```python
from build123d import *

# Parameters (mm, degrees)
EXTRUDE_1_DEPTH = 3
FILLET_1_R      = 2.032


with BuildPart() as part:
    # 스케치1 → 보스-돌출1 (new body)
    with BuildSketch(Plane.XY):
        with BuildLine():
            Line((-22.703212056, -30.53470544), (-22.703212056, -27.53470544))
            Line((-22.703212056, -27.53470544), (-19.808212056, -27.53470544))
            Line((-19.808212056, -27.53470544), (-19.808212056, -30.53470544))
            ThreePointArc((-19.808212056, -30.53470544), (-17.458089238, -27.052134486), (-19.755712056, -23.53470544))
            ThreePointArc((-19.755712056, -23.53470544), (-16.806747664, -15.831278272), (-10.426669431, -10.603106234))
            ThreePointArc((-10.426669431, -10.603106234), (-4.615473218, -6.174719455), (-1.296316018, 0.334028993))
            ThreePointArc((-1.296316018, 0.334028993), (-1.766656874, 1.136185733), (-2.575803416, 0.677974178))
            ThreePointArc((-2.575803416, 0.677974178), (-5.721510813, -5.168139004), (-11.025821999, -9.160230838))
            ThreePointArc((-11.025821999, -9.160230838), (-18.562919164, -14.982954912), (-22.755712056, -23.53470544))
            ThreePointArc((-22.755712056, -23.53470544), (-25.053334873, -27.052134486), (-22.703212056, -30.53470544))
        make_face()
    extrude(amount=EXTRUDE_1_DEPTH)

    # 필렛1
    fillet_1_edges = [part.edges().sort_by_distance(p)[0] for p in [
        (-22.755712056, -23.53470544, 1.5),
        (-19.755712056, -23.53470544, 1.5),
    ]]
    fillet(fillet_1_edges, radius=FILLET_1_R)


solid = part.part
```
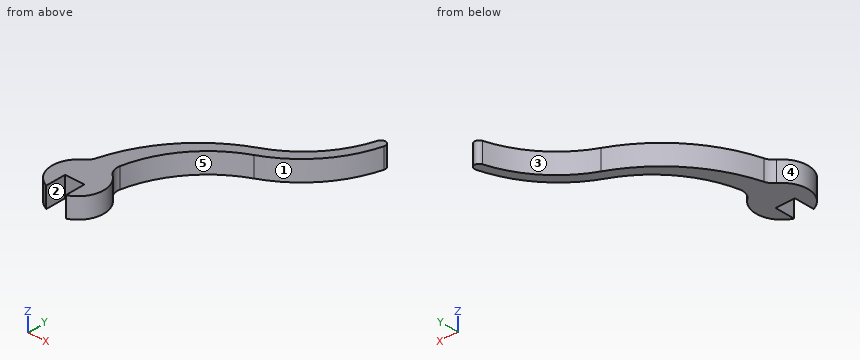
The model under review builds one solid part; all positions refer to its coordinate system, in mm. Face numbers are marked on the shaded views. A direction names the side the tool comes from. Round coordinates to 2 decimals unless told otherwise and drop trailing zeros. Order: outer loops, then holes, each group sorted by start corner. A loop starts at its lowest first (then second) coordinate and runs counter-clockwise, first axis right, second up. Notation, with made-up numbers: (89.5, 39.5) -> (142.5, 39.5) arc R16 ccw to (142.5, 70.5) -> close; hole circle Ø1 at (36, 76). An arc over 180 degrees is marked (long way). One line per item, written item: value. Start each with the question number.
Q1. Wall thickness on line 1 (Y direction, x = -17.75, z = 1.5); line 2 (Y direction, x = -18, z = 1.25); line 3 (X direction, y = -10, z = 2.05): over which ranges is each line inside the solid? List them lowest first.
Q2. Machinability: for the marked faces 4 and 5, which of the approach directions +Z, -Z, +X, -X, +Y, -Y give a long, thin tool a straight path to every point of the face, cutting with its end or side? Answer none if there is none.
Q3. Clearance check with flat-ended pins moving along their axes: pin 1 Ø0.9 at (y, z) = (-28.5, 2) entering from -X; pin 2 Ø1 at (x, z) = (-4.5, 2.5) entering from -Y; pin 3 Ø1 at (y, z) = (-12.5, 2) entering from +X; pin 4 Ø10 at (x, y) = (-16, -20.5) entering from -Z. State where each tip first meets the part, or that it passes through.
Q4. Take a section at C-C (x = -4). Write out the cut boundary in (y, z), and give its area (3 significant figures).
Q5. Mouldability with a two-part tool opening along X and no side actions: class the marked faces 1, 2 and 3 as released by +X, released by -X, zero draft, split by the parting line, or undercut.
Q6. Take a section at A-A (x = -18.25). Write out the cut boundary in (y, z).
Q7. Take a section at B-B (y = -5.5). Write out the cut boundary in (x, z), and give its area (3 significant figures).
Reported:
1. line 1: y = -28.48 to -25.56, -17.3 to -14.04
1. line 2: y = -28.98 to -25.07, -17.76 to -14.32
1. line 3: x = -12.67 to -9.23
2. face 4: +Z, -Z, -X
2. face 5: +Z, -Z, +X
3. pin 1: stops at x = -24.91
3. pin 2: stops at y = -6.62
3. pin 3: stops at x = -12.89
3. pin 4: stops at z = 0
4. outline: (-5.39, 0) -> (-2.72, 0) -> (-2.72, 3) -> (-5.39, 3) -> close
4. area: 8.01 mm2
5. face 1: released by +X
5. face 2: undercut
5. face 3: released by -X
6. outline: (-29.34, 0) -> (-24.7, 0) -> (-24.7, 3) -> (-29.34, 3) -> close; (-18.25, 0) -> (-14.61, 0) -> (-14.61, 3) -> (-18.25, 3) -> close
7. outline: (-6.01, 0) -> (-4.08, 0) -> (-4.08, 3) -> (-6.01, 3) -> close
7. area: 5.80 mm2
